Check sheet for the modelled part. Datum: model origin and axes. Units: mm. A direction names the side the tool comes from. Coordinates: 2 decimals unless noted, no trailing zeros. Write each loop counter-clockwise with the first axis right and the second up, starting at its lowest first coordinate (ties: lowest second). Pieces come first, ordered by that corner, then holes. Notation, with made-up numbers: M -11.75,3 L 46.25,3 A24 cw 46.25,19 Z; hole C 10.25,29.5 d8. An arc over 180 degrees is marked long. Answer as CSV lines item,"result".
from build123d import *

# Parameters (mm, degrees)
F0_R     = 2
F1_DEPTH = 3


with BuildPart() as f1:
    # F0 (on Front) → F1 (new body)
    with BuildSketch(Plane.XZ):
        with BuildLine():
            Line((-7.5, 24), (-7.5, -55))
            ThreePointArc((-7.5, -55), (0, -62.5), (7.5, -55))
            Line((7.5, -55), (7.5, 24))
            ThreePointArc((7.5, 24), (0, 31.5), (-7.5, 24))
        make_face()
        Circle(F0_R, mode=Mode.SUBTRACT)
        with BuildLine():
            ThreePointArc((-1, 24), (0, 25), (1, 24))
            Line((1, 24), (1, 4))
            ThreePointArc((1, 4), (0, 3), (-1, 4))
            Line((-1, 4), (-1, 24))
        make_face(mode=Mode.SUBTRACT)
    extrude(amount=F1_DEPTH)


solid = f1.part
1) Thickness scan on line 1 along Z through (x, y) = (0, -1.95); line 2 along X through (y, z) = (-1.9, 18.5); line 3 along X through (y, z) = (-1.85, -55.5). Record the ranges inside material, lowest first.
Answer key:
line 1,"z = -62.5 to -2, 2 to 3, 25 to 31.5"
line 2,"x = -7.5 to -1, 1 to 7.5"
line 3,"x = -7.48 to 7.48"
2) Section check B-B, the plane x = 0. Record the boundary of the cut face in (y, z), plus the area to 3 significant figures.
Answer key:
outline,"M -3,-62.5 L 0,-62.5 L 0,-2 L -3,-2 Z; M -3,2 L 0,2 L 0,3 L -3,3 Z; M -3,25 L 0,25 L 0,31.5 L -3,31.5 Z"
area,"204 mm2"
3) Section check C-C, the plane y = -1.85. Record the boundary of the cut face in (x, z).
Answer key:
outline,"M -7.5,-55 A7.5 ccw 7.5,-55 L 7.5,24 A7.5 ccw -7.5,24 Z; hole C 0,0 d4; hole M -1,4 A1 ccw 1,4 L 1,24 A1 ccw -1,24 Z"
4) Section check D-D, the plane z = 12. Record the boundary of the cut face in (x, y), plus the area to 3 significant figures.
Answer key:
outline,"M -7.5,-3 L -1,-3 L -1,0 L -7.5,0 Z; M 1,-3 L 7.5,-3 L 7.5,0 L 1,0 Z"
area,"39.0 mm2"
5) Tool access check on faces 4 (the face through (7.5, -1, -16)), 5 (the face through (1, -1, 14)). Record the directions out of +Z, -Z, +X, -X, +Y, -Y that give a thin tool (end or side, any length) a straight path to the whole face; none if there is none.
Answer key:
face 4,"+Z, -Z, +X, +Y, -Y"
face 5,"+Y, -Y"
6) Mould release check, pull along X, two halves, no side actions. Record for faces 1 (the face through (0.16, -1.48, 31.5)), 2 (the face through (-7.5, -1, -15)), 3 (the face through (0, -1, 25)): pulls with the +X half, pulls with the -X half, needs draft (parallel to the pull), parting line crosses it, or undercut.
Answer key:
face 1,"parting line crosses it"
face 2,"pulls with the -X half"
face 3,"undercut"
7) Section check A-A, the plane z = 0. Record the boundary of the cut face in (x, y).
Answer key:
outline,"M -7.5,-3 L -2,-3 L -2,0 L -7.5,0 Z; M 2,-3 L 7.5,-3 L 7.5,0 L 2,0 Z"
